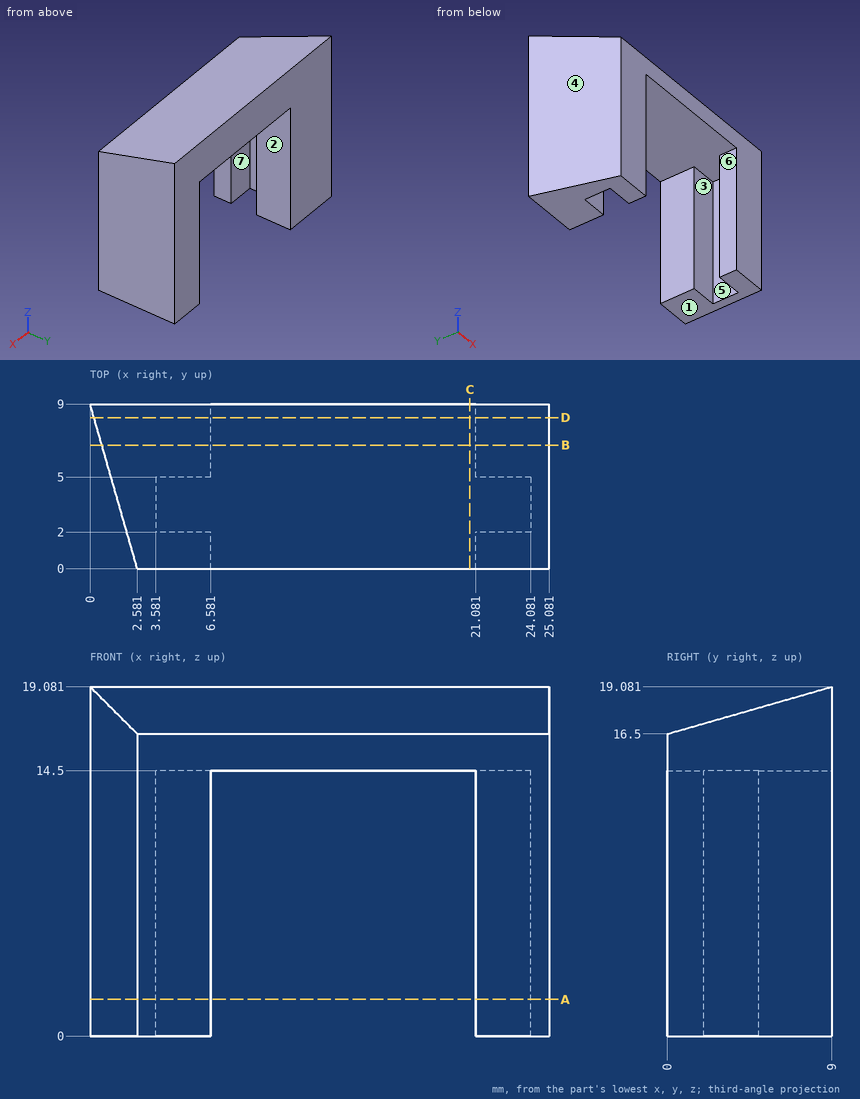
Study the drawing (mm; zero at the part's minimum x, y, z) and answer. A direction names the side the tool comes from. Coordinates: 2 decimals unless noted, no trailing zeros. Write each loop counter-clockwise with the first axis right and the second up, starting at its lowest first coordinate (ties: lowest second). Pieces come first, ordered by that corner, then holes. Notation, with made-up numbers: (58.25, 52) - (109.25, 52) arc R17 cw to (109.25, 77) - close; hole circle Ø10 at (-28, -16.75). An arc over 180 degrees is marked (long way). Answer as a JSON object with one key per item and string values.
Q1. Find section B-B (y = 6.75). Write down the section's boundary in (x, z) (1 decimal).
Results list:
{"outline": "(0.6, 0) - (6.6, 0) - (6.6, 14.5) - (21.1, 14.5) - (21.1, 0) - (25.1, 0) - (25.1, 18.4) - (0.6, 18.4) - close"}
Q2. Consider L1, parallel to Y at x = 22.75, z = 13.5; L2, parallel to X at y = 4.75, z = 14; L3, parallel to X at y = 4.5, z = 6. Determine where each line is inside the solid, lowest interval first. Write a range as from..to.
Results list:
{"L1": "y = 0..2, 5..9", "L2": "x = 1.22..3.58, 24.08..25.08", "L3": "x = 1.29..3.58, 24.08..25.08"}
Q3. Which of the six approach directions +Z, -Z, +X, -X, +Y, -Y give full straight-line access (tool end or side, diameter ignored) to the marked faces 1, 2 and 3?
Results list:
{"face 1": "-Z, +X, -X, +Y, -Y", "face 2": "-Z, +Y, -Y", "face 3": "-Z"}
Q4. For a pull along Y with two mould halves and no side action, classify the marked faces 4, 5, 6 and 7 as pulls with the +Y half, pulls with the -Y half, needs draft (parallel to the pull), parting line crosses it, or undercut.
Results list:
{"face 4": "pulls with the -Y half", "face 5": "undercut", "face 6": "needs draft", "face 7": "undercut"}
Q5. Find section C-C (x = 20.75). Write down the section's boundary in (y, z).
Results list:
{"outline": "(0, 14.5) - (9, 14.5) - (9, 19.08) - (0, 16.5) - close"}
Q6. Given pin 1 Ø2 at (y, z) = (7.5, 5) entering from -X; pin 2 Ø2 at (y, z) = (1, 9.5) entering from -X; pin 3 Ø2.5 at (y, z) = (3, 10.5) entering from -X, each flat-ended and moving along its own axis, determine where each tip first touches the part or whether it passes through.
Results list:
{"pin 1": "stops at x = 0.14", "pin 2": "stops at x = 2.01", "pin 3": "stops at x = 1.36"}
Q7. Find section D-D (y = 8.25). Write down the section's boundary in (x, z) (1 decimal).
Results list:
{"outline": "(0.2, 0) - (6.6, 0) - (6.6, 14.5) - (21.1, 14.5) - (21.1, 0) - (25.1, 0) - (25.1, 18.9) - (0.2, 18.9) - close"}
Q8. Find section A-A (z = 2). Write down the section's boundary in (x, y).
Results list:
{"outline": "(0, 9) - (2.58, 0) - (6.58, 0) - (6.58, 2) - (3.58, 2) - (3.58, 5) - (6.58, 5) - (6.58, 9) - close; (21.08, 0) - (25.08, 0) - (25.08, 9) - (21.08, 9) - (21.08, 5) - (24.08, 5) - (24.08, 2) - (21.08, 2) - close"}
